Design review of the part built by this model. Coordinates are the model's own, in mm. Coordinates: 2 decimals unless noted, no trailing zeros. Order: outer loops, then holes, each group sorted by start corner. A loop starts at its lowest first (then second) coordinate and runs counter-clockwise, first axis right, second up. Notation, with made-up numbers: M -14,-6 L 8,-6 A22 ccw 8,18 Z; hole C 68.5,-33 d1. An arc over 180 degrees is marked long. Use CSV: the item, a comma, the result in double quotes.
```python
from build123d import *

# Parameters (mm, degrees)
SKETCH3_R               = 3.175
BOSS_EXTRUDE1_DEPTH     = 304.8
CHAMFER1_SIZE           = 0.635
CUT_EXTRUDE1_START      = -118.327050112
SKETCH4_R               = 3.175
CUT_EXTRUDE1_DEPTH      = 492.272949888
SKETCH5_R               = 0.5953125
CUT_EXTRUDE2_DEPTH      = 4.175
CUT_EXTRUDE2_DEPTH_BACK = 4.175


with BuildPart() as part:
    # Sketch3 → Boss-Extrude1 (new body, symmetric)
    with BuildSketch(Plane.XY):
        Circle(SKETCH3_R)
    extrude(amount=BOSS_EXTRUDE1_DEPTH, both=True)

    # Chamfer1
    chamfer1_edges = [part.edges().sort_by_distance(p)[0] for p in [
        (-3.175, 0, -304.8),
        (-3.175, 0, 304.8),
    ]]
    chamfer(chamfer1_edges, length=CHAMFER1_SIZE)

    # Sketch4 → Cut-Extrude1 (cut, through all)
    with BuildSketch(Plane.XY.offset(304.8).offset(CUT_EXTRUDE1_START)):
        Circle(SKETCH4_R)
    extrude(amount=-CUT_EXTRUDE1_DEPTH, mode=Mode.SUBTRACT)

    # Sketch5 → Cut-Extrude2 (cut, two sides)
    with BuildSketch(Plane(origin=(0, 0, 0), x_dir=(1, 0, 0), z_dir=(0, 1, 0))) as cut_extrude2_sk:
        with Locations((0, -188.060449888)):
            Circle(SKETCH5_R)
        with Locations((0, -303.2125)):
            Circle(SKETCH5_R)
    extrude(amount=CUT_EXTRUDE2_DEPTH, mode=Mode.SUBTRACT)
    extrude(cut_extrude2_sk.sketch, amount=-CUT_EXTRUDE2_DEPTH_BACK, mode=Mode.SUBTRACT)


solid = part.part
```
(1) Clearance check with flat-ended pins moving along their axes: P1, Ø0.7, axis at x = 0, z = 303.21, coming from the -Y side; P2, Ø2, axis at x = 0.5, z = 282, coming from the +Y side (3 decimals); P3, Ø1, axis at x = 1.5, z = 290, coming from the -Y side. State where each tip first meets the part, or that it passes through.
The answers:
P1,"passes through"
P2,"stops at y = 3.175"
P3,"stops at y = -3.01"
(2) Add section A-A on y = -1. Give the number of separate pieces and of enclosed holes in the cut face, and give its area (3 significant figures).
The answers:
separate pieces,"1"
enclosed holes,"2"
area,"710 mm2"
(3) Wall thickness on probe 1 along Z at (x, y) = (0, 1.6); probe 2 along Z at (x, y) = (-0.5, 2.25); probe 3 along Y at (x, z) = (-0.25, 209): over which ranges is each line inside the solid? List them lowest first.
The answers:
probe 1,"z = 186.47 to 187.47, 188.66 to 302.62, 303.81 to 304.8"
probe 2,"z = 186.47 to 187.74, 188.38 to 302.89, 303.54 to 304.8"
probe 3,"y = -3.17 to 3.17"
(4) Add section B-B on z = 247.5. State the section outline as (x, y) points (3 decimals).
The answers:
outline,"C 0,0 d6.35"
